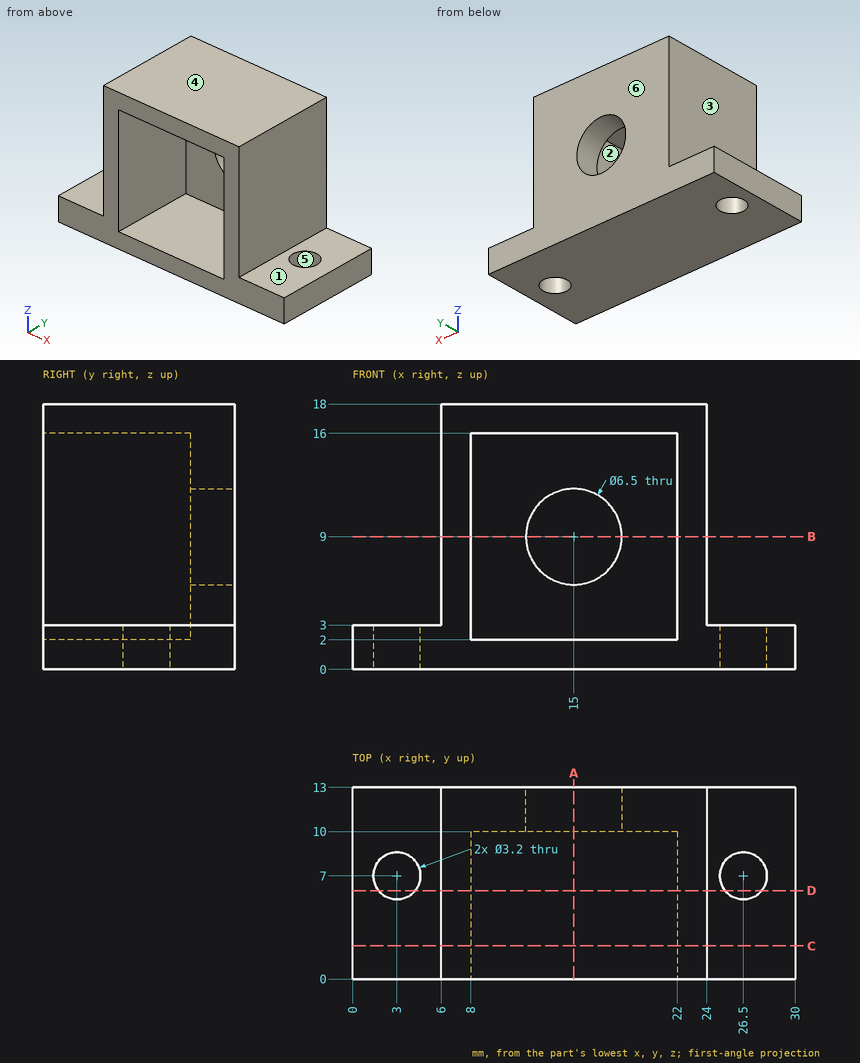
Could you check a few things on this drawing? It's one solid part, dimensions in mm from its lowest x, y, z. A direction names the side the tool comes from. Give positions to 0.01 mm unless a question says otherwise; leave off trailing zeros. Write each loop counter-clockwise with the first axis right and the second up, starting at its lowest first coordinate (ties: lowest second). Pieces come first, ordered by that corner, then holes. Notation, with made-up numbers: (17, -34) -> (43, -34) arc R30 cw to (43, 1) -> close; hole circle Ø7 at (54, 22). An arc over 180 degrees is marked (long way). Answer as a JSON object with one key per item and string values.
Q1. Will these pins go through, and if not, where does the flat tip stop? pin 1 Ø5 at (x, y) = (2.5, 5.5) entering from +Z; pin 2 Ø4 at (y, z) = (9.5, 11.5) entering from +X; pin 3 Ø6.5 at (y, z) = (3.5, 9.5) entering from -X.
Taken from the geometry:
{"pin 1": "stops at z = 3", "pin 2": "stops at x = 24", "pin 3": "stops at x = 6"}
Q2. Suppose I cut it at D-D on y = 6. Write out the boundary of the cut face in (x, z), then the cut area to 3 significant figures.
Taken from the geometry:
{"outline": "(0, 0) -> (1.75, 0) -> (1.75, 3) -> (0, 3) -> close; (4.25, 0) -> (25.25, 0) -> (25.25, 3) -> (24, 3) -> (24, 18) -> (6, 18) -> (6, 3) -> (4.25, 3) -> close; (27.75, 0) -> (30, 0) -> (30, 3) -> (27.75, 3) -> close; hole (8, 2) -> (22, 2) -> (22, 16) -> (8, 16) -> close", "area": "149 mm²"}
Q3. Please list where these lines run through material, in increasing order: L1, parallel to X at y = 7, z = 2.4; L2, parallel to Y at x = 3, z = 1.75; L3, parallel to Z at x = 14.75, y = 7.75.
Taken from the geometry:
{"L1": "x = 0 to 1.4, 4.6 to 8, 22 to 24.9, 28.1 to 30", "L2": "y = 0 to 5.4, 8.6 to 13", "L3": "z = 0 to 2, 16 to 18"}
Q4. Suppose I cut it at A-A on x = 15. Write out the boundary of the cut face in (y, z).
Taken from the geometry:
{"outline": "(0, 0) -> (13, 0) -> (13, 5.75) -> (10, 5.75) -> (10, 2) -> (0, 2) -> close; (0, 16) -> (10, 16) -> (10, 12.25) -> (13, 12.25) -> (13, 18) -> (0, 18) -> close"}
Q5. Suppose I cut it at B-B on z = 9. Write out the boundary of the cut face in (x, y).
Taken from the geometry:
{"outline": "(6, 0) -> (8, 0) -> (8, 10) -> (11.75, 10) -> (11.75, 13) -> (6, 13) -> close; (18.25, 10) -> (22, 10) -> (22, 0) -> (24, 0) -> (24, 13) -> (18.25, 13) -> close"}
Q6. Suppose I cut it at C-C on y = 2.25. Write out the boundary of the cut face in (x, z).
Taken from the geometry:
{"outline": "(0, 0) -> (30, 0) -> (30, 3) -> (24, 3) -> (24, 18) -> (6, 18) -> (6, 3) -> (0, 3) -> close; hole (8, 2) -> (22, 2) -> (22, 16) -> (8, 16) -> close"}
Q7. Which directions (+Z, -Z, +X, -X, +Y, -Y) give clear straight access to the entire face, cutting with the end or side of a thin tool? Please do the marked faces 1, 2 and 3.
Taken from the geometry:
{"face 1": "+Z, +X, +Y, -Y", "face 2": "-Y", "face 3": "+Z, -X, +Y, -Y"}
Q8. We'd pull the mould along Y, two halves only. Please class the marked faces 4, 5 and 6: released by +Y, released by -Y, zero draft, split by the parting line, or undercut.
Taken from the geometry:
{"face 4": "zero draft", "face 5": "undercut", "face 6": "released by +Y"}
